Geometry check sheet. Reference: the model listing, model coordinates, mm. Face numbers are marked on the shaded views. A direction names the side the tool comes from. Round coordinates to 2 decimals unless told otherwise and drop trailing zeros. Write each loop counter-clockwise with the first axis right and the second up, starting at its lowest first coordinate (ties: lowest second). Pieces come first, ordered by that corner, then holes.
Item 1: Cross-section at C-C (y = 1.25). Enter the section's corners in (x, z).
Item 2: Draft check along X on the marked faces 3, 4 and 5. Enter one of: pulls with the +X half, pulls with the -X half, needs draft (parallel to the pull), parting line crosses it, or undercut.
Item 3: Cross-section at B-B (x = 0). Enter the section's corners in (y, z), then the cut area to 3 significant figures.
Item 4: Scan lines: probe 1 along X at (y, z) = (7.25, 0); probe 2 along Y at (x, z) = (43.7, 0); probe 3 along Z at (x, y) = (-7, 1). Record each from-to range of solid material in increasing order.
Item 5: Access from +Z, -Z, +X, -X, +Y, -Y to the whole of each face (thin tool, end or side, straight path). Record for the marked faces 1 and 2.
Item 6: Cross-section at A-A (z = 0). Enter the section's corners in (x, y).
Item 7: Depth check by flat-ended pin: P1, Ø2.5, axis at y = 4.5, z = -2.5, coming from the +X side; P2, Ø4, axis at y = 7, z = -10.5, coming from the -X side; P3, Ø3.5, axis at y = 5, z = -0.5, coming from the -X side. Enter the tip coordinate at first touch or a pass-through.
Item 8: Cross-section at D-D (z = 12.5). Enter the section's corners in (x, y), then the cut area to 3 significant figures.
from build123d import *

# Parameters (mm, degrees)
SKETCH1_R               = 50
SKETCH1_R_2             = 42.5
BOSS_EXTRUDE1_DEPTH     = 9
BOSS_EXTRUDE2_START     = -9
BOSS_EXTRUDE2_DEPTH     = 9
CUT_EXTRUDE1_DEPTH      = 89
CUT_EXTRUDE1_DEPTH_BACK = 5
SKETCH3_R               = 1.5


with BuildPart() as part:
    # Sketch1 → Boss-Extrude1 (new body)
    with BuildSketch(Plane(origin=(0, 0, 0), x_dir=(1, 0, 0), z_dir=(0, 1, 0))):
        with Locations(Location((0, 0, 0), (0, 0, 270))):
            Circle(SKETCH1_R)
        with Locations(Location((0, 0, 0), (0, 0, 270))):
            Circle(SKETCH1_R_2, mode=Mode.SUBTRACT)
    extrude(amount=BOSS_EXTRUDE1_DEPTH)

    # Sketch2 → Boss-Extrude2 (add)
    with BuildSketch(Plane(origin=(0, 9, 0), x_dir=(1, 0, 0), z_dir=(0, 1, 0)).offset(BOSS_EXTRUDE2_START)):
        with BuildLine():
            ThreePointArc((-42, 6.5), (-42.5, 0), (-42, -6.5))
            Line((-42, -6.5), (-42, 6.5))
        make_face()
        with BuildLine():
            Line((42, 6.5), (42, -6.5))
            ThreePointArc((42, -6.5), (42.374815634, -3.259601203), (42.5, 0))
            ThreePointArc((42.5, 0), (42.374815634, 3.259601203), (42, 6.5))
        make_face()
    extrude(amount=BOSS_EXTRUDE2_DEPTH)

    # Sketch3 → Cut-Extrude1 (cut, two sides: drawn at the far end of the back side and taken through both)
    with BuildSketch(Plane(origin=(-42, 0, 0), x_dir=(0, 0, -1), z_dir=(1, 0, 0)).offset(-CUT_EXTRUDE1_DEPTH_BACK)):
        with Locations((0, 4.5)):
            Circle(SKETCH3_R)
    extrude(amount=CUT_EXTRUDE1_DEPTH + CUT_EXTRUDE1_DEPTH_BACK, mode=Mode.SUBTRACT)


solid = part.part
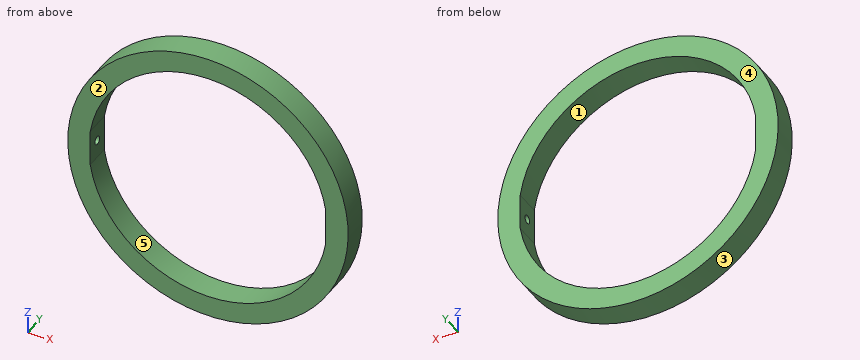
Resolved:
1. outline: circle Ø100 at (0, 0); hole (-42, -6.5) arc R42.5 ccw to (42, -6.5) - (42, 6.5) arc R42.5 ccw to (-42, 6.5) - close
2. face 3: parting line crosses it
2. face 4: needs draft
2. face 5: undercut
3. outline: (0, -50) - (9, -50) - (9, -42.5) - (0, -42.5) - close; (0, 42.5) - (9, 42.5) - (9, 50) - (0, 50) - close
3. area: 135 mm2
4. probe 1: x = -50 to -42, 42 to 50
4. probe 2: y = 0 to 3, 6 to 9
4. probe 3: z = -49.51 to -41.92, 41.92 to 49.51
5. face 1: +Y, -Y
5. face 2: +Z, -Z, +X, -X, -Y
6. outline: (-50, 0) - (-42, 0) - (-42, 3) - (-47, 3) - (-47, 6) - (-42, 6) - (-42, 9) - (-50, 9) - close; (42, 0) - (50, 0) - (50, 9) - (42, 9) - (42, 6) - (47, 6) - (47, 3) - (42, 3) - close
7. P1: stops at x = 49.98
7. P2: stops at x = -49.27
7. P3: stops at x = -50
8. outline: (-48.41, 0) - (-40.62, 0) - (-40.62, 9) - (-48.41, 9) - close; (40.62, 0) - (48.41, 0) - (48.41, 9) - (40.62, 9) - close
8. area: 140 mm2
